Design review of the part built by this model. Coordinates are the model's own, in mm. Coordinates: 2 decimals unless noted, no trailing zeros. Loops run counter-clockwise (first coordinate to the right, second up) from the corner with the lowest first, then second, coordinate; pieces in that order, holes last. Notation, with made-up numbers: (8, 26.25) -> (32, 26.25) arc R20 cw to (32, 65.25) -> close; hole circle Ø7 at (-13, 56.5). An arc over 180 degrees is marked (long way). One line per item, written item: value. Start each with the question number.
1. Add section D-D on x = 53. Write out the cut boundary in (y, z), plus the area to 3 significant figures.
2. For probe 1 along Y at (x, z) = (48, 0.4); probe 2 along Y at (x, z) = (-43, 0.55); probe 3 along X at (y, z) = (-31, 0.8), list the stretches that pass through material, from the lowest coordinate up.
3. Add section A-A on y = 0. Write out the cut boundary in (x, z), plus the area to 3 significant figures.
4. Insertion check: pin 1 (6 mm diameter, centred on x = -54.5, y = 33.5, fed in from -Z). The pin has a flat end and moves straight along its axis. Give the tip position at first contact, or say it passes through.
5. Add section B-B on x = 0. Write out the cut boundary in (y, z), plus the area to 3 significant figures.
6. Add section C-C on y = 44. Write out the cut boundary in (x, z), plus the area to 3 significant figures.
```python
from build123d import *

# Parameters (mm, degrees)
ESBO_O1_R                = 25
ESBO_O1_R_2              = 20
RESSALTO_EXTRUS_O1_DEPTH = 1
ESBO_O2_R                = 4
CORTE_EXTRUS_O1_DEPTH    = 1


with BuildPart() as part:
    # Esboço1 → Ressalto-extrusão1 (new body)
    with BuildSketch(Plane.XY):
        with BuildLine():
            Line((-46, -75.019997334), (46, -75.019997334))
            ThreePointArc((46, -75.019997334), (0, 88), (-46, -75.019997334))
        make_face()
        Circle(ESBO_O1_R, mode=Mode.SUBTRACT)
        with Locations((-35, 54.772)):
            Circle(ESBO_O1_R_2, mode=Mode.SUBTRACT)
        with Locations((35, 54.772)):
            Circle(ESBO_O1_R_2, mode=Mode.SUBTRACT)
        with Locations((-54.772, -35)):
            Circle(ESBO_O1_R_2, mode=Mode.SUBTRACT)
        with Locations((54.772, -35)):
            Circle(ESBO_O1_R_2, mode=Mode.SUBTRACT)
    extrude(amount=RESSALTO_EXTRUS_O1_DEPTH)

    # Esboço2 → Corte-extrusão1 (cut)
    with BuildSketch(Plane.XY.offset(1)):
        with Locations((81.5, 0)):
            Circle(ESBO_O2_R)
        with Locations((-81.5, 0)):
            Circle(ESBO_O2_R)
    extrude(amount=-CORTE_EXTRUS_O1_DEPTH, mode=Mode.SUBTRACT)


solid = part.part
```
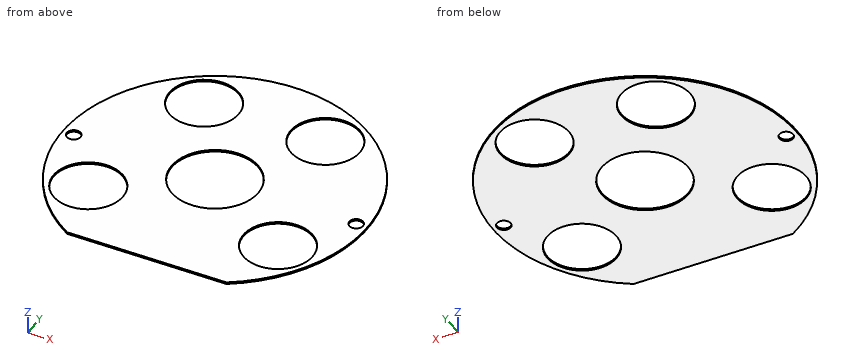
Worked answers:
1. outline: (-70.25, 0) -> (-54.92, 0) -> (-54.92, 1) -> (-70.25, 1) -> close; (-15.08, 0) -> (46.05, 0) -> (46.05, 1) -> (-15.08, 1) -> close; (63.49, 0) -> (70.25, 0) -> (70.25, 1) -> (63.49, 1) -> close
1. area: 83.2 mm²
2. probe 1: y = -73.76 to -53.82, -16.18 to 39.57, 69.97 to 73.76
2. probe 2: y = -75.02 to -51.17, -18.83 to 36.44, 73.1 to 76.78
2. probe 3: x = -82.36 to -74.37, -35.18 to 35.18, 74.37 to 82.36
3. outline: (-88, 0) -> (-85.5, 0) -> (-85.5, 1) -> (-88, 1) -> close; (-77.5, 0) -> (-25, 0) -> (-25, 1) -> (-77.5, 1) -> close; (25, 0) -> (77.5, 0) -> (77.5, 1) -> (25, 1) -> close; (85.5, 0) -> (88, 0) -> (88, 1) -> (85.5, 1) -> close
3. area: 110 mm²
4. pin 1: stops at z = 0
5. outline: (-75.02, 0) -> (-25, 0) -> (-25, 1) -> (-75.02, 1) -> close; (25, 0) -> (88, 0) -> (88, 1) -> (25, 1) -> close
5. area: 113 mm²
6. outline: (-76.21, 0) -> (-51.85, 0) -> (-51.85, 1) -> (-76.21, 1) -> close; (-18.15, 0) -> (18.15, 0) -> (18.15, 1) -> (-18.15, 1) -> close; (51.85, 0) -> (76.21, 0) -> (76.21, 1) -> (51.85, 1) -> close
6. area: 85.0 mm²
